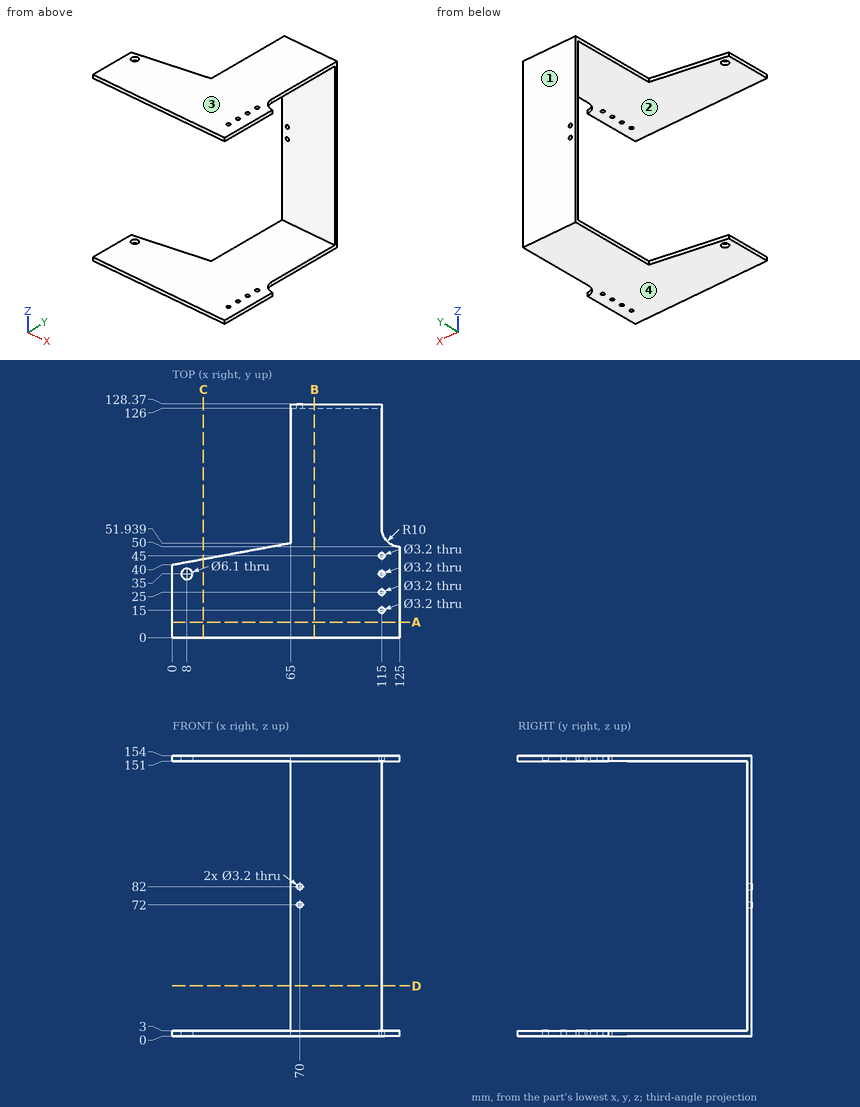
Here's the drawing with two shaded views (mm, measured from the low corner). I have some questions. Coordinates: 2 decimals unless noted, no trailing zeros. Order: outer loops, then holes, each group sorted by start corner. A loop starts at its lowest first (then second) coordinate and runs counter-clockwise, first axis right, second up.
Q1. Suppose I cut it at B-B on x = 78. Please give me the cut outline in (y, z), and give its area (3 significant figures).
Q2. Thinking about a two-plate mould opening in Z: for the marked faces 1, 2, 3 and 4, which applies, released by +Z, released by -Z, zero draft, split by the parting line, or undercut?
Q3. Will these pins go through, and if not, where does the flat tip stop? pin 1 (1.9 mm diameter, centred on x = 115, y = 25, fed in from -Z); pin 2 (2 mm diameter, centred on x = 110, z = 45.5, fed in from -Y).
Q4. Please list where these lines run through material, in increasing order: L1, parallel to X at y = 25, z = 152; L2, parallel to Z at x = 79.5, y = 24; L3, parallel to Z at x = 70, y = 127.
Q5. Suppose I cut it at D-D on z = 27.5. Please give me the cut outline in (x, y).
Q6. Suppose I cut it at C-C on x = 17. Please give me the cut outline in (y, z), and give its area (3 significant figures).
Q7. Suppose I cut it at A-A on y = 8.5. Please give me the cut outline in (x, z), and give its area (3 significant figures).
Answer:
1. outline: (0, 0) - (128.37, 0) - (128.37, 154) - (0, 154) - (0, 151) - (126, 151) - (126, 3) - (0, 3) - close
1. area: 1,120 mm2
2. face 1: zero draft
2. face 2: undercut
2. face 3: released by +Z
2. face 4: released by -Z
3. pin 1: passes through
3. pin 2: stops at y = 126
4. L1: x = 0 to 113.4, 116.6 to 125
4. L2: z = 0 to 3, 151 to 154
4. L3: z = 0 to 70.4, 73.6 to 80.4, 83.6 to 154
5. outline: (65, 126) - (115, 126) - (115, 128.37) - (65, 128.37) - close
6. outline: (0, 0) - (43.12, 0) - (43.12, 3) - (0, 3) - close; (0, 151) - (43.12, 151) - (43.12, 154) - (0, 154) - close
6. area: 259 mm2
7. outline: (0, 0) - (125, 0) - (125, 3) - (0, 3) - close; (0, 151) - (125, 151) - (125, 154) - (0, 154) - close
7. area: 750 mm2
